Input: part model. Units: mm. Frame: model coordinates. A direction names the side the tool comes from. Coordinates: 2 decimals unless noted, no trailing zeros. Order: outer loops, then holes, each group sorted by start corner. A loop starts at its lowest first (then second) coordinate and runs counter-clockwise, first axis right, second up. Notation, with made-up numbers: M 55,33 L 74,33 A7 ccw 74,43 Z; hole C -27.5,-26.5 d10. An arc over 180 degrees is marked long. Answer in a Markdown table with one row per item.
from build123d import *

# Parameters (mm, degrees)
BASPROSKE_W             = 10
BASPROSKE_H             = 8
TOOTHCUT_DEPTH          = 16.099668871
TEETHCUTS_COUNT         = 14
TEETHCUTS_ANGLE         = 334.285714286
BORSKE_R                = 0.5
BORE_DEPTH              = 50.0000508
CUT_EXTRUDE1_DEPTH      = 16.017018917
CUT_EXTRUDE2_DEPTH      = 16.017018917
CUT_EXTRUDE2_DEPTH_BACK = 16.017018917
SKETCH2_R               = 3.75


with BuildPart() as part:
    # BasProSke → Base-Revolve (revolve)
    with BuildSketch(Plane(origin=(0, 0, 0), x_dir=(1, 0, 0), z_dir=(0, 1, 0)), mode=Mode.PRIVATE) as base_revolve_sk:
        with Locations((5, 4)):
            Rectangle(BASPROSKE_W, BASPROSKE_H)
    revolve(base_revolve_sk.sketch.rotate(Axis((-10, 0, 0), (1, 0, 0)), 180), axis=Axis((-10, 0, 0), (1, 0, 0)))

    # TooCutSke → ToothCut (cut, through all)
    with BuildSketch(Plane(origin=(0, 0, 0), x_dir=(0, 0, -1), z_dir=(1, 0, 0))):
        with BuildLine():
            ThreePointArc((0.540393256, 5.723545765), (0, 5.749), (-0.540393256, 5.723545765))
            ThreePointArc((-0.540393256, 5.723545765), (-0.832220085, 6.912663993), (-1.603550271, 7.863566092))
            ThreePointArc((-1.603550271, 7.863566092), (0, 8.0254), (1.603550271, 7.863566092))
            ThreePointArc((1.603550271, 7.863566092), (0.832220085, 6.912663993), (0.540393256, 5.723545765))
        make_face()
    toothcut = extrude(amount=TOOTHCUT_DEPTH, mode=Mode.SUBTRACT)

    # TeethCuts: ToothCut ×14 about axis
    teethcuts_axis = Axis((-10, 0, 0), (1, 0, 0))
    for i in range(1, TEETHCUTS_COUNT):
        add(toothcut.rotate(teethcuts_axis, i * TEETHCUTS_ANGLE / (TEETHCUTS_COUNT - 1)), mode=Mode.SUBTRACT)

    # BorSke → Bore (cut, symmetric)
    with BuildSketch(Plane(origin=(0, 0, 0), x_dir=(0, 0, -1), z_dir=(1, 0, 0))):
        with Locations(Location((0, 0, 0), (0, 0, 180))):
            Circle(BORSKE_R)
    extrude(amount=BORE_DEPTH, both=True, mode=Mode.SUBTRACT)

    # Sketch1 → Cut-Extrude1 (cut, through all)
    with BuildSketch(Plane(origin=(10, 0, 0), x_dir=(0, 0, -1), z_dir=(1, 0, 0))):
        Polygon((-1.125, -1.125), (-1.125, -3.375), (1.125, -3.375), (1.125, -1.125), (3.375, -1.125), (3.375, 1.125), (1.125, 1.125), (1.125, 3.375), (-1.125, 3.375), (-1.125, 1.125), (-3.375, 1.125), (-3.375, -1.125), align=None)
    extrude(amount=-CUT_EXTRUDE1_DEPTH, mode=Mode.SUBTRACT)

    # Sketch2 → Cut-Extrude2 (cut, two sides: drawn at the far end of the back side and taken through both)
    with BuildSketch(Plane(origin=(10, 0, 0), x_dir=(0, 0, -1), z_dir=(1, 0, 0)).offset(-CUT_EXTRUDE2_DEPTH_BACK)):
        Circle(SKETCH2_R)
    extrude(amount=CUT_EXTRUDE2_DEPTH + CUT_EXTRUDE2_DEPTH_BACK, mode=Mode.SUBTRACT)


solid = part.part
1) Contact query for flat-ended pins moving along their axis: pin 1 (4 mm diameter, centred on x = 4, y = 4.5, fed in from +Z); pin 2 (1.5 mm diameter, centred on y = -5, z = -6, fed in from +X); pin 3 (1.5 mm diameter, centred on x = 7, z = -4.5, fed in from +Y). Output: stop coordinate, or through.
Resolved:
| item | result |
|---|---|
| pin 1 | stops at z = 7.3 |
| pin 2 | passes through |
| pin 3 | stops at y = 6.38 |
2) Cut plane B-B, the plane y = 0. Output: boundary loops of the cut face in (x, z), and give its area (3 significant figures).
Resolved:
| item | result |
|---|---|
| outline | M 0,-8 L 10,-8 L 10,-3.75 L 0,-3.75 Z; M 0,3.75 L 10,3.75 L 10,8 L 0,8 Z |
| area | 85.0 mm2 |
3) Cut plane A-A, the plane z = 0. Output: boundary loops of the cut face in (x, y), and give its area (3 significant figures).
Resolved:
| item | result |
|---|---|
| outline | M 0,-5.75 L 10,-5.75 L 10,-3.75 L 0,-3.75 Z; M 0,3.75 L 10,3.75 L 10,5.75 L 0,5.75 Z |
| area | 40.0 mm2 |
4) Material intervals for probe 1 along Z at (x, y) = (4.5, 0); probe 2 along Y at (x, z) = (7.5, 0); probe 3 along Y at (x, z) = (7.75, -7), sorted ascending.
Resolved:
| item | result |
|---|---|
| probe 1 | z = -8 to -3.75, 3.75 to 8 |
| probe 2 | y = -5.75 to -3.75, 3.75 to 5.75 |
| probe 3 | y = -3.68 to -2.81, -0.71 to 0.71, 2.81 to 3.68 |
5) Reachability of faces 1 (the face through (4.93, 5.846, 3.723)), 2 (the face through (4.93, -5.87, 3.75)), 3 (the face through (4.93, -3.59, -4.49)) from +Z, -Z, +X, -X, +Y, -Y: full face, straight path, thin tool, end or side. Return the list, or none.
Resolved:
| item | result |
|---|---|
| face 1 | +X, -X, +Y |
| face 2 | +X, -X, -Y |
| face 3 | +X, -X |
6) Mould query, pull axis Z, two halves, no side actions, for faces 4 (the face through (4.93, 2.35, 6.555)), 5 (the face through (4.93, -0.735, -6.892)). Classes: +Z half, -Z half, draft (parallel to the pull), parting line (faces both ways), or undercut.
Resolved:
| item | result |
|---|---|
| face 4 | +Z half |
| face 5 | undercut |
